For this review, take the finished solid that the model builds, in its own axes (mm). Face numbers are marked on the shaded views. Round coordinates to 2 decimals unless told otherwise and drop trailing zeros. Write each loop counter-clockwise with the first axis right and the second up, starting at its lowest first coordinate (ties: lowest second). Pieces come first, ordered by that corner, then holes. Notation, with made-up numbers: M -8.5,47 L 40.5,47 A24 cw 40.5,63 Z; hole C 26.25,68 d8. An arc over 180 degrees is marked long. One line per question, with ' | ' between items.
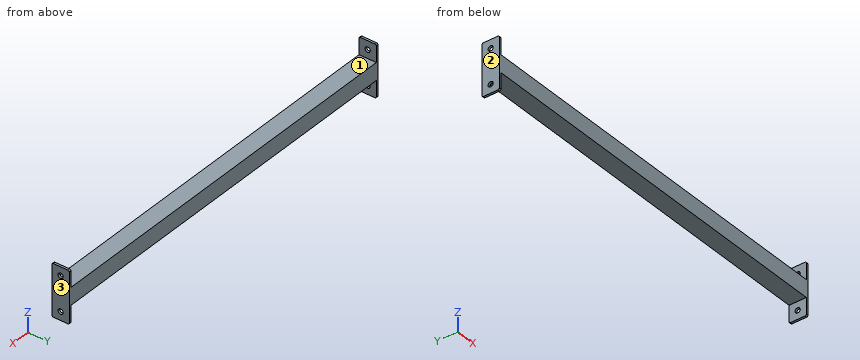
```python
from build123d import *

# Parameters (mm, degrees)
F0_W     = 40
F0_H     = 40
F0_W_2   = 35
F0_H_2   = 35
F1_DEPTH = 450
F2_R     = 6
F3_DEPTH = 5


with BuildPart() as f1:
    # F0 (on Right) → F1 (new body, symmetric)
    with BuildSketch(Plane.YZ):
        Rectangle(F0_W, F0_H)
        Rectangle(F0_W_2, F0_H_2, mode=Mode.SUBTRACT)
    extrude(amount=F1_DEPTH, both=True)

    # F2 (on face) → F3 (join)
    with BuildSketch(Plane.YZ.offset(450)):
        with BuildLine():
            Line((20, -20), (20, 20))
            Line((20, 20), (-20, 20))
            Line((-20, 20), (-20, -20))
            Line((-20, -20), (-20, -57))
            ThreePointArc((-20, -57), (-19.1213203436, -59.1213203436), (-17, -60))
            Line((-17, -60), (17, -60))
            ThreePointArc((17, -60), (19.1213203436, -59.1213203436), (20, -57))
            Line((20, -57), (20, -20))
        make_face()
        with Locations((0, -40)):
            Circle(F2_R, mode=Mode.SUBTRACT)
        with BuildLine():
            Line((-20, 20), (20, 20))
            Line((20, 20), (20, 57))
            ThreePointArc((20, 57), (19.1213203436, 59.1213203436), (17, 60))
            Line((17, 60), (-17, 60))
            ThreePointArc((-17, 60), (-19.1213203436, 59.1213203436), (-20, 57))
            Line((-20, 57), (-20, 20))
        make_face()
        with Locations((0, 40)):
            Circle(F2_R, mode=Mode.SUBTRACT)
    extrude(amount=F3_DEPTH)

    # F4: F1 across plane


with BuildPart() as f1_1:
    add(f1.part)
    add(f1.part.mirror(Plane.YZ))


solid = f1_1.part
```
Item 1: Take a section at B-B (x = -279). Write out the cut boundary in (y, z), then the cut area to 3 significant figures.
Results:
outline: M -20,-20 L 20,-20 L 20,20 L -20,20 Z; hole M -17.5,-17.5 L 17.5,-17.5 L 17.5,17.5 L -17.5,17.5 Z | area: 375 mm2
Item 2: Insertion check: pin 1 Ø8 at (x, y) = (133.5, 3) entering from -Z; pin 2 Ø20 at (x, y) = (33.5, 8) entering from +Z. Each pin has a flat end and moves straight along its axis. Give the tip position at first contact, or say it passes through.
Results:
pin 1: z = -20 | pin 2: z = 20
Item 3: Mouldability with a two-part tool opening along X and no side actions: class the marked faces 1, 2 and 3 as +X half, -X half, draft (parallel to the pull), parting line (faces both ways), or undercut.
Results:
face 1: undercut | face 2: -X half | face 3: +X half
Item 4: To check wall thickness, follow line 1 along Z through (x, y) = (-452.6, 0); line 2 along Z through (x, y) = (352, 5.5); line 3 along X through (y, z) = (-12, 8.5). State the ranges of each line that lie inside material, in increasing order. Write a range as from..to.
Results:
line 1: -60..-46, -34..34, 46..60 | line 2: -20..-17.5, 17.5..20 | line 3: -455..-450, 450..455
Item 5: Take a section at A-A (z = 7.5). Write out the cut boundary in (x, y).
Results:
outline: M -455,-20 L 455,-20 L 455,20 L -455,20 Z; hole M -450,-17.5 L 450,-17.5 L 450,17.5 L -450,17.5 Z
